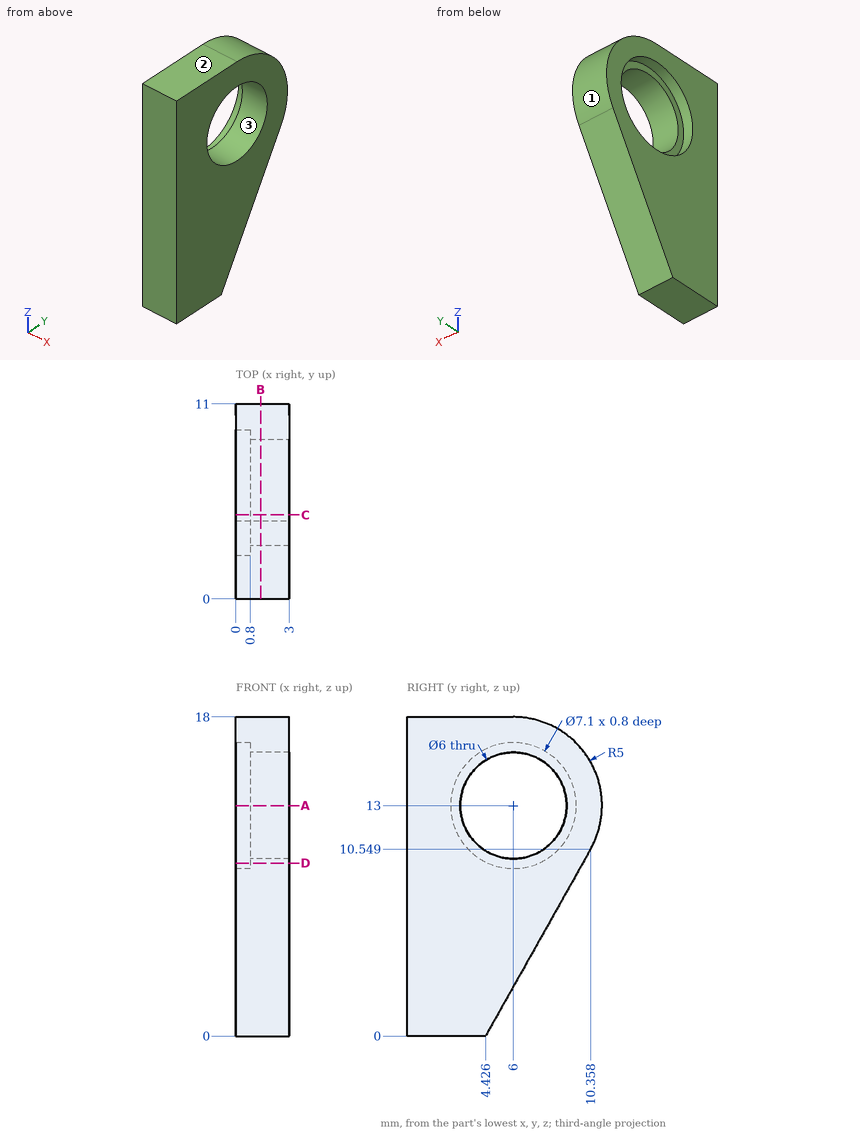
The drawing under review shows one solid part. Ordinate dimensions are in mm from its lowest x, y, z. Give positions to 0.01 mm unless a question says otherwise; leave off trailing zeros. Order: outer loops, then holes, each group sorted by start corner. A loop starts at its lowest first (then second) coordinate and runs counter-clockwise, first axis right, second up. Notation, with made-up numbers: (61.25, -32.75) -> (119.25, -32.75) arc R33 ccw to (119.25, 0.25) -> close; hole circle Ø1 at (24, 50). An arc over 180 degrees is marked (long way). Write item = value, one per line.
1) We need section A-A, the plane z = 13. Give the boundary of the cut face in (x, y).
Findings:
outline = (0, 0) -> (3, 0) -> (3, 3) -> (0.8, 3) -> (0.8, 2.45) -> (0, 2.45) -> close; (0, 9.55) -> (0.8, 9.55) -> (0.8, 9) -> (3, 9) -> (3, 11) -> (0, 11) -> close
2) Draft analysis for pull direction Y (two halves, no side actions). For the marked faces 1, 2 and 3, state which applies: pulls with the +Y half, pulls with the -Y half, needs draft (parallel to the pull), parting line crosses it, or undercut.
Findings:
face_1 = pulls with the +Y half
face_2 = needs draft
face_3 = undercut
3) We need section C-C, the plane y = 4.75. Give the boundary of the cut face in (x, z).
Findings:
outline = (0, 0.58) -> (3, 0.58) -> (3, 10.27) -> (0.8, 10.27) -> (0.8, 9.68) -> (0, 9.68) -> close; (0, 16.32) -> (0.8, 16.32) -> (0.8, 15.73) -> (3, 15.73) -> (3, 18) -> (0, 18) -> close
4) Insertion check: pin 1 (1 mm diameter, centred on x = 0.5, z = 15.5, fed in from +Y); pin 2 (5.5 mm diameter, centred on y = 5.5, z = 13.5, fed in from -X). Each pin has a flat end and moves straight along its axis. Give the tip position at first contact, or say it passes through.
Findings:
pin_1 = 10.58
pin_2 = 0.8
5) We need section D-D, the plane z = 9.75. Give the boundary of the cut face in (x, y).
Findings:
outline = (0, 0) -> (3, 0) -> (3, 9.91) -> (0, 9.91) -> (0, 7.43) -> (0.8, 7.43) -> (0.8, 4.57) -> (0, 4.57) -> close
6) To check wall thickness, follow L1, parallel to Y at x = 2.4, z = 13; L2, parallel to Y at x = 1.95, z = 15.75 (1 decimal); L3, parallel to Z at x = 0.2, y = 5 (1 decimal). State the ranges of each line that lie inside material, in increasing order. Write a range as from..to.
Findings:
L1 = 0..3, 9..11
L2 = 0..4.8, 7.2..10.2
L3 = 1..9.6, 16.4..18
7) We need section B-B, the plane x = 1.4. Give the boundary of the cut face in (y, z).
Findings:
outline = (0, 0) -> (4.43, 0) -> (10.36, 10.55) arc R5 ccw to (6, 18) -> (0, 18) -> close; hole circle Ø6 at (6, 13)
